For this review, take the finished solid that the model builds, in its own axes (mm). A direction names the side the tool comes from. Coordinates: 2 decimals unless noted, no trailing zeros. Loops run counter-clockwise (first coordinate to the right, second up) from the corner with the lowest first, then second, coordinate; pieces in that order, holes last. Notation, with made-up numbers: M 39,-27 L 93,-27 A11 cw 93,-11 Z; hole C -11,52 d4. An arc over 180 degrees is marked long. Use one line per item in the form item = value.
```python
from build123d import *
from OCP.BRepFilletAPI import BRepFilletAPI_MakeChamfer

# Parameters (mm, degrees)
BOSS_EXTRUDE1_DEPTH = 15
CHAMFER1_SIZE       = 8
CHAMFER1_SIZE2      = 11.425184054


with BuildPart() as part:
    # Sketch1 → Boss-Extrude1 (new body)
    with BuildSketch(Plane.XY):
        Polygon((34.047005384, 58.97114317), (-34.047005384, 58.97114317), (-68.094010768, 0), (-34.047005384, -58.97114317), (34.047005384, -58.97114317), (68.094010768, 0), align=None)
        Polygon((45, 0), (22.5, 38.97114317), (-22.5, 38.97114317), (-45, 0), (-22.5, -38.97114317), (22.5, -38.97114317), align=None, mode=Mode.SUBTRACT)
    extrude(amount=BOSS_EXTRUDE1_DEPTH)

    # Chamfer1: one chamfer whose edges measure the first distance from different faces: ONE call of the kernel's chamfer builder (chamfer() names one face for all edges)
    chamfer1_edges_1 = [part.edges().sort_by_distance(p)[0] for p in [
        (-51.070508076, -29.485571585, 15),
    ]]
    chamfer1_side_1 = [part.faces().sort_by_distance(p)[0] for p in [
        (-51.070508076, -29.485571585, 7.5),
    ]]
    chamfer1_edges_2 = [part.edges().sort_by_distance(p)[0] for p in [
        (51.070508076, -29.485571585, 15),
    ]]
    chamfer1_side_2 = [part.faces().sort_by_distance(p)[0] for p in [
        (51.070508076, -29.485571585, 7.5),
    ]]
    chamfer1_edges_3 = [part.edges().sort_by_distance(p)[0] for p in [
        (0, 58.97114317, 15),
    ]]
    chamfer1_side_3 = [part.faces().sort_by_distance(p)[0] for p in [
        (0, 58.97114317, 7.5),
    ]]
    chamfer1 = BRepFilletAPI_MakeChamfer(part.part.solid().wrapped)
    for e in chamfer1_edges_1:
        chamfer1.Add(CHAMFER1_SIZE, CHAMFER1_SIZE2, e.wrapped, chamfer1_side_1[0].wrapped)  # the first distance lies on this face
    for e in chamfer1_edges_2:
        chamfer1.Add(CHAMFER1_SIZE, CHAMFER1_SIZE2, e.wrapped, chamfer1_side_2[0].wrapped)  # the first distance lies on this face
    for e in chamfer1_edges_3:
        chamfer1.Add(CHAMFER1_SIZE, CHAMFER1_SIZE2, e.wrapped, chamfer1_side_3[0].wrapped)  # the first distance lies on this face
    add(Compound.cast(chamfer1.Shape()), mode=Mode.REPLACE)


solid = part.part
```
1. Consider section A-A on x = -5.5. Write out the cut boundary in (y, z).
Computed values:
outline = M -58.97,0 L -38.97,0 L -38.97,15 L -58.97,15 Z; M 38.97,0 L 58.97,0 L 58.97,7 L 47.55,15 L 38.97,15 Z
2. Wall thickness on line 1 along Y through (x, z) = (-10, 4.75); line 2 along X through (y, z) = (-23.5, 12); line 3 along X through (y, z) = (-31, 8): over which ranges is each line inside the solid? List them lowest first. Write a range as from..to.
Computed values:
line_1 = -58.97..-38.97, 38.97..58.97
line_2 = -46.28..-31.43, 31.43..46.28
line_3 = -48.55..-27.1, 27.1..48.55
3. Tool access review of faces 1 (the face through (-1, 40, 0)), 2 (the face through (0, -38.971, 7)): name each direction out of +Z, -Z, +X, -X, +Y, -Y from which nothing blocks a thin tool from reaching the whole face with its end or side.
Computed values:
face_1 = -Z, +X, -X, +Y, -Y
face_2 = +Z, -Z
4. Consider section C-C on y = 3.5. Write out the cut boundary in (x, z), plus the area to 3 significant figures.
Computed values:
outline = M -66.07,0 L -42.98,0 L -42.98,15 L -56.92,15 L -66.07,9.45 Z; M 42.98,0 L 66.07,0 L 66.07,9.45 L 56.92,15 L 42.98,15 Z
area = 642 mm2
5. Consider section B-B on z = 5. Write out the cut boundary in (x, y), plus the area to 3 significant figures.
Computed values:
outline = M -68.09,0 L -34.05,-58.97 L 34.05,-58.97 L 68.09,0 L 34.05,58.97 L -34.05,58.97 Z; hole M -45,0 L -22.5,-38.97 L 22.5,-38.97 L 45,0 L 22.5,38.97 L -22.5,38.97 Z
area = 6,790 mm2
6. Consider section D-D on x = 31. Write out the cut boundary in (y, z).
Computed values:
outline = M -58.97,0 L -24.25,0 L -24.25,15 L -41.4,15 L -58.97,8.85 Z; M 24.25,0 L 58.97,0 L 58.97,7 L 47.55,15 L 24.25,15 Z
7. Draft analysis for pull direction X (two halves, no side actions). For faces 3 (the face through (-46.339, -26.097, 11.056)), 4 (the face through (33.91, 19.21, 7.4)), 5 (the face through (-37, 18, 15)), state which applies: +X half, -X half, draft (parallel to the pull), parting line (faces both ways), or undercut.
Computed values:
face_3 = -X half
face_4 = undercut
face_5 = draft
8. For pin 1 Ø1.5 at (y, z) = (-22.5, 10.5) entering from -X; pin 2 Ø2 at (y, z) = (30.5, 5) entering from +X; pin 3 Ø8 at (x, z) = (-38, 8.5) entering from +Y, all flat-tipped, find the tip position at first contact; note any pin that passes through.
Computed values:
pin_1 = -50.64
pin_2 = 51.06
pin_3 = 58.68
